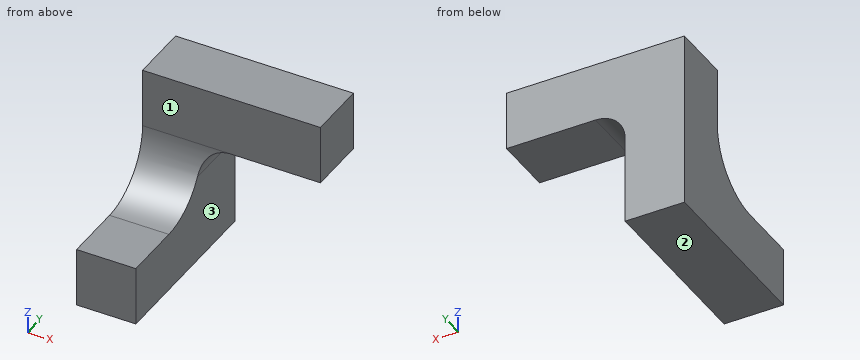
from build123d import *

# Parameters (mm, degrees)
F1_DEPTH = 76.2
F3_DEPTH = 76.201


with BuildPart() as f1:
    # F0 (on Front) → F1 (new body)
    with BuildSketch(Plane.XZ):
        with BuildLine():
            Line((0, 76.2), (0, 0))
            Line((0, 0), (25.4, 0))
            Line((25.4, 0), (25.4, 38.1))
            ThreePointArc((25.4, 38.1), (29.119744, 47.080256), (38.1, 50.8))
            Line((38.1, 50.8), (76.2, 50.8))
            Line((76.2, 50.8), (76.2, 76.2))
            Line((76.2, 76.2), (0, 76.2))
        make_face()
    extrude(amount=F1_DEPTH)

    # F2 (on face) → F3 (cut, through all)
    with BuildSketch(Plane.YZ.offset(76.2)):
        with BuildLine():
            Line((-76.2, 76.2), (-76.2, 25.4))
            Line((-76.2, 25.4), (-50.8, 25.4))
            ThreePointArc((-50.8, 25.4), (-32.839488, 32.839488), (-25.4, 50.8))
            Line((-25.4, 50.8), (-25.4, 76.2))
            Line((-25.4, 76.2), (-76.2, 76.2))
        make_face()
    extrude(amount=-F3_DEPTH, mode=Mode.SUBTRACT)


solid = f1.part
Here's how the part is built. I have some questions about the finished solid (model axes, mm). Face numbers are marked on the shaded views. A direction names the side the tool comes from. Round coordinates to 2 decimals unless told otherwise and drop trailing zeros. Order: outer loops, then holes, each group sorted by start corner. A loop starts at its lowest first (then second) coordinate and runs counter-clockwise, first axis right, second up. Notation, with made-up numbers: M 1.5,47.5 L 58.5,47.5 A24 cw 58.5,80.5 Z; hole C 50,-11.75 d3. An arc over 180 degrees is marked long. Return JSON: item names as keys, results as strings. Group by question number.
1. I'm going to push flat-ended pins straight in: pin 1 Ø10 at (y, z) = (-44, 13.5) entering from +X; pin 2 Ø7.5 at (x, y) = (56, -7) entering from -Z; pin 3 Ø3 at (y, z) = (-40.5, 30) entering from -X; pin 4 Ø7.5 at (x, y) = (9, -66.5) entering from +Z. Where does each tip first touch, or does it pass through?
2. If we section it at A-A on x = 14: List the corners of the cut face in (y, z) for me, then the cut area to 3 significant figures.
3. If we section it at B-B on y = -11.5: List the corners of the cut face in (x, z) for me.
4. Please list where these lines run through material, in increasing order: probe 1 along X at (y, z) = (-61, 11); probe 2 along Z at (x, y) = (47, -18); probe 3 along Y at (x, z) = (71, 52.5).
5. If we section it at C-C on z = 23: List the corners of the cut face in (x, y) for me.
6. If we section it at D-D on x = 51: List the corners of the cut face in (y, z) for me, then the cut area to 3 significant figures.
7. On a 3-axis mill with a long thin cutter (end or side, diameter ignored), from which of +Z, -Z, +X, -X, +Y, -Y can I reach the whole of each face in a straight line? I mean the marked faces 1, 2 and 3. Say none if no direction works.
Reply:
{
 "1": {"pin 1": "x = 25.4", "pin 2": "z = 50.8", "pin 3": "through", "pin 4": "z = 25.4"},
 "2": {"outline": "M -76.2,0 L 0,0 L 0,76.2 L -25.4,76.2 L -25.4,50.8 A25.4 cw -50.8,25.4 L -76.2,25.4 Z", "area": "3,360 mm^2"},
 "3": {"outline": "M 0,0 L 25.4,0 L 25.4,38.1 A12.7 cw 38.1,50.8 L 76.2,50.8 L 76.2,76.2 L 0,76.2 Z"},
 "4": {"probe 1": "0 to 25.4", "probe 2": "50.8 to 76.2", "probe 3": "-25.4 to 0"},
 "5": {"outline": "M 0,-76.2 L 25.4,-76.2 L 25.4,0 L 0,0 Z"},
 "6": {"outline": "M -25.4,50.8 L 0,50.8 L 0,76.2 L -25.4,76.2 Z", "area": "645 mm^2"},
 "7": {"face 1": "+Z, +X, -X, -Y", "face 2": "-Z, +X, -X, +Y, -Y", "face 3": "-Z, +X, +Y, -Y"}
}
